Could you check a few things on this drawing? It's one solid part, dimensions in mm from its lowest x, y, z. Coordinates: 2 decimals unless noted, no trailing zeros. Write each loop counter-clockwise with the first axis right and the second up, starting at its lowest first coordinate (ties: lowest second). Pieces come first, ordered by that corner, then holes. Notation, with made-up numbers: (17.25, 5) - (31.25, 5) arc R23 ccw to (31.25, 23) - close; hole circle Ø9 at (-9, 36). An arc over 180 degrees is marked (long way). Use one line per item in the form item = value. Start each with the question number.
(1) For pin 1 Ø5 at (x, y) = (60, 6) entering from -Z; pin 2 Ø3.5 at (x, y) = (60, 6) entering from -Z, each with a flat end and sliding along its axis, tell me the tip position at first contact or that it passes through.
(2) If we section it at A-A on z = 174: Please give me the cut outline in (x, y), then the cut area to 4 significant figures.
(3) If I drill on probe 1 along X at (y, z) = (6, 181.25); probe 2 along Y at (x, z) = (10, 8); probe 3 along X at (y, z) = (7.25, 180), over which ranges is the centre line in solid material (lowest first)? Write a range as from..to.
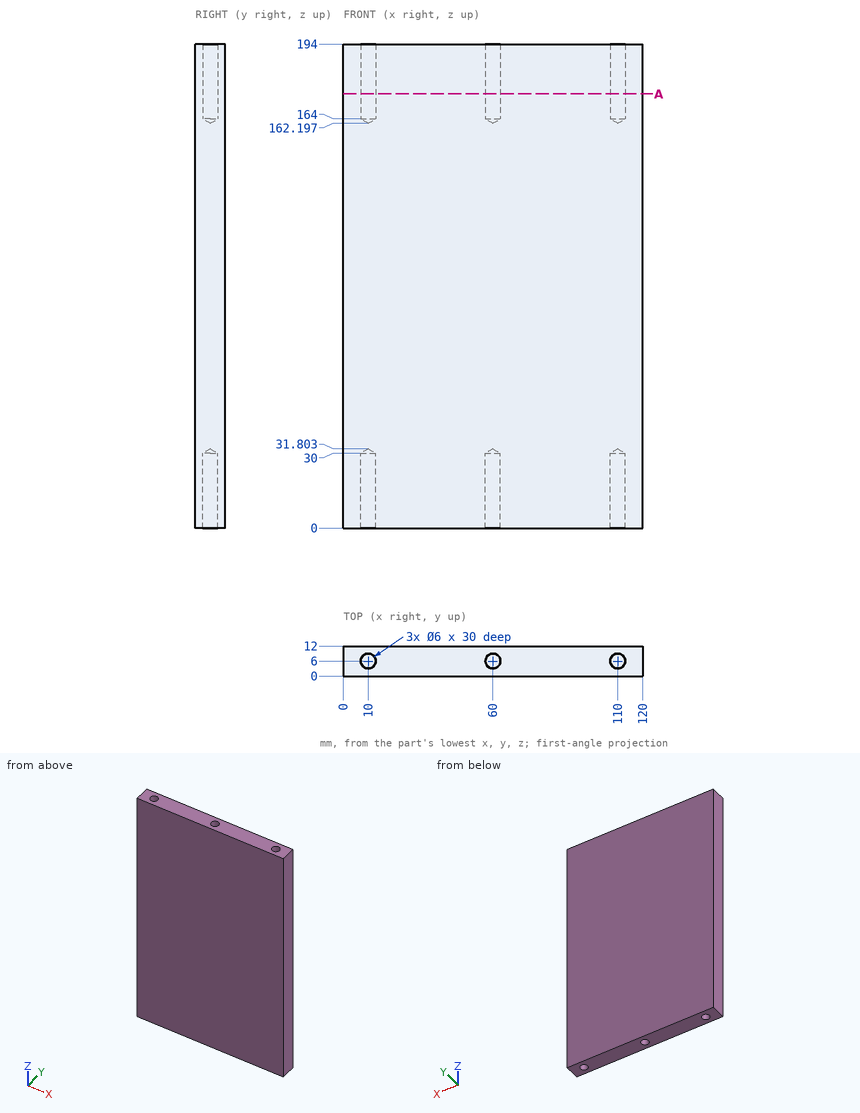
Reported:
q1.pin_1 = 30.3
q1.pin_2 = 30.75
q2.outline = (0, 0) - (120, 0) - (120, 12) - (0, 12) - close; hole circle Ø6 at (10, 6); hole circle Ø6 at (60, 6); hole circle Ø6 at (110, 6)
q2.area = 1,355 mm2
q3.probe_1 = 0..7, 13..57, 63..107, 113..120
q3.probe_2 = 0..3, 9..12
q3.probe_3 = 0..7.27, 12.73..57.27, 62.73..107.27, 112.73..120
